```python
from build123d import *

# Parameters (mm, degrees)
F0_W     = 38.1
F0_H     = 19.05
F1_DEPTH = 2.54
F2_R     = 1.016
F3_DEPTH = 10.16
F4_DEPTH = 10.16


# Not quite as in the source:
# - a feature names something its author has since deleted; it is built from what else it names


with BuildPart() as f1:
    # F0 (on Front) → F1 (new body)
    with BuildSketch(Plane.XZ):
        Rectangle(F0_W, F0_H)
    extrude(amount=F1_DEPTH)

    # F2 (on face) → F3 (join)
    with BuildSketch(Plane.XZ.offset(2.54)):
        with Locations((-14.9520980194, 5.6684408337)):
            Circle(F2_R)
        with Locations((-8.8560991403, 5.6721375078)):
            Circle(F2_R)
        with Locations((-8.8793454933, 2.1162134919)):
            Circle(F2_R)
        with Locations((-14.9753443725, 2.1125168178)):
            Circle(F2_R)
        with Locations((-14.9985907255, -1.4434071982)):
            Circle(F2_R)
        with Locations((-8.9025918464, -1.439710524)):
            Circle(F2_R)
        with Locations((-8.9258381994, -4.99563454)):
            Circle(F2_R)
        with Locations((-15.0218370786, -4.9993312141)):
            Circle(F2_R)
        with Locations((-2.8298393203, -4.9919378658)):
            Circle(F2_R)
        with Locations((-2.8065929672, -1.4360138499)):
            Circle(F2_R)
        with Locations((-2.7833466142, 2.119910166)):
            Circle(F2_R)
        with Locations((-2.7601002611, 5.675834182)):
            Circle(F2_R)
        with Locations((3.335898618, 5.6795308561)):
            Circle(F2_R)
        with Locations((3.312652265, 2.1236068402)):
            Circle(F2_R)
        with Locations((3.2894059119, -1.4323171757)):
            Circle(F2_R)
        with Locations((3.2661595589, -4.9882411917)):
            Circle(F2_R)
    extrude(amount=F3_DEPTH)

    # F2 (on face) → F4 (join)
    with BuildSketch(Plane.XZ.offset(2.54)):
        with Locations((9.4318974972, 5.6832275303)):
            Circle(F2_R)
        with Locations((9.4086511441, 2.1273035143)):
            Circle(F2_R)
        with Locations((9.3854047911, -1.4286205016)):
            Circle(F2_R)
        with Locations((9.362158438, -4.9845445175)):
            Circle(F2_R)
        with Locations((15.4581573172, -4.9808478434)):
            Circle(F2_R)
        with Locations((15.4814036702, -1.4249238275)):
            Circle(F2_R)
        with Locations((15.5046500233, 2.1310001885)):
            Circle(F2_R)
        with Locations((15.5278963763, 5.6869242044)):
            Circle(F2_R)
    extrude(amount=F4_DEPTH)


solid = f1.part
```
Geometry check sheet. Reference: the model listing, model coordinates, mm. A direction names the side the tool comes from. Round coordinates to 2 decimals unless told otherwise and drop trailing zeros. Loops run counter-clockwise (first coordinate to the right, second up) from the corner with the lowest first, then second, coordinate; pieces in that order, holes last. Notation, with made-up numbers: M -14.5,20.5 L -3.5,20.5 A13 cw -3.5,42.5 Z; hole C -22.75,-10.5 d6. An arc over 180 degrees is marked long. Return JSON: item names as keys, results as strings. Group by question number.
(1) Section check C-C, the plane z = 1.5. Enter the section's corners in (x, y), and give its area (3 significant figures).
(2) Go/stop test with flat-tipped pins: pin 1 (1 mm diameter, centred on x = -10, y = -6, fed in from -Z); pin 2 (3 mm diameter, centred on x = -3.5, y = -9, fed in from +Z). Record where each tip stops, or that it passes through.
(3) Scan lines: line 1 along Z through (x, y) = (2.5, -11.25); line 2 along X through (y, z) = (-5.5, 2.75); line 3 along Z through (x, y) = (16, -10). Record each from-to range of solid material in increasing order. Write a range as [from, to].
(4) Section check A-A, the plane y = -7. Give the number of separate pieces and of enclosed holes in the cut face, and give its area (3 significant figures).
(5) Mould release check, pull along Z, two halves, no side actions. Record for faces 3 (the face through (3.18, -7.55, 3.13)), 4 (the face through (9, -12.7, -5)), 5 (the face through (0, -1, 9.525)): pulls with the +Z half, pulls with the -Z half, needs draft (parallel to the pull), parting line crosses it, or undercut.
(6) Section check B-B, the plane x = -15.5. Enter the section's corners in (y, z) (3 decimals), and give its area (3 significant figures).
(7) Section check D-D, the plane x = 9. Enter the section's corners in (y, z) (1 decimal), and give its area (3 significant figures).
(8) Set-up check for faces 1 (the face through (-15, -12.7, -1)), 2 (the face through (10.301, -7.549, -5.374)): record each of +Z, -Z, +X, -X, +Y, -Y from which the full face is reachable in a straight line by a thin tool's end or side.
Data:
{
 "1": {"outline": "M -19.05,-2.54 L -15.79,-2.54 L -15.79,-12.7 L -14.16,-12.7 L -14.16,-2.54 L -9.69,-2.54 L -9.69,-12.7 L -8.07,-12.7 L -8.07,-2.54 L -3.59,-2.54 L -3.59,-12.7 L -1.98,-12.7 L -1.98,-2.54 L 2.51,-2.54 L 2.51,-12.7 L 4.11,-12.7 L 4.11,-2.54 L 8.61,-2.54 L 8.61,-12.7 L 10.21,-12.7 L 10.21,-2.54 L 14.71,-2.54 L 14.71,-12.7 L 16.3,-12.7 L 16.3,-2.54 L 19.05,-2.54 L 19.05,0 L -19.05,0 Z", "area": "195 mm²"},
 "2": {"pin 1": "z = -5.83", "pin 2": "z = 6.69"},
 "3": {"line 1": "[-5.66, -4.32], [-2.07, -0.79], [1.51, 2.73], [5.1, 6.26]", "line 2": "[-15.77, -14.18], [-9.67, -8.09], [-3.58, -1.99], [2.51, 4.11], [8.61, 10.21], [14.7, 16.31]", "line 3": "[-5.84, -4.12], [-2.3, -0.55], [1.24, 3.02], [4.79, 6.59]"},
 "4": {"separate pieces": "24", "enclosed holes": "0", "area": "77.8 mm²"},
 "5": {"face 3": "undercut", "face 4": "needs draft", "face 5": "pulls with the +Z half"},
 "6": {"outline": "M -12.7,-5.896 L -2.54,-5.896 L -2.54,-9.525 L 0,-9.525 L 0,9.525 L -2.54,9.525 L -2.54,6.524 L -12.7,6.524 L -12.7,4.813 L -2.54,4.813 L -2.54,2.983 L -12.7,2.983 L -12.7,1.242 L -2.54,1.242 L -2.54,-0.56 L -12.7,-0.56 L -12.7,-2.327 L -2.54,-2.327 L -2.54,-4.103 L -12.7,-4.103 Z", "area": "120 mm²"},
 "7": {"outline": "M -12.7,-5.9 L -2.5,-5.9 L -2.5,-9.5 L 0,-9.5 L 0,9.5 L -2.5,9.5 L -2.5,6.6 L -12.7,6.6 L -12.7,4.8 L -2.5,4.8 L -2.5,3.1 L -12.7,3.1 L -12.7,1.2 L -2.5,1.2 L -2.5,-0.5 L -12.7,-0.5 L -12.7,-2.4 L -2.5,-2.4 L -2.5,-4 L -12.7,-4 Z", "area": "124 mm²"},
 "8": {"face 1": "+Z, -Z, +X, -X, -Y", "face 2": "-Y"}
}
